from build123d import *

# Parameters (mm, degrees)
SKETCH1_R           = 2.1
BOSS_EXTRUDE1_DEPTH = 50


with BuildPart() as part:
    # Sketch1 → Boss-Extrude1 (new body)
    with BuildSketch(Plane(origin=(0, 0, 0), x_dir=(0, 0, -1), z_dir=(1, 0, 0))):
        with BuildLine():
            Line((-13, 18), (-13, 20))
            Line((-13, 20), (-19, 20))
            ThreePointArc((-19, 20), (-19.707106781, 19.707106781), (-20, 19))
            Line((-20, 19), (-20, 13))
            Line((-20, 13), (-18, 13))
            Line((-18, 13), (-18, 16))
            Line((-18, 16), (-17.060660172, 16))
            Line((-17.060660172, 16), (-14, 12.939339828))
            Line((-14, 12.939339828), (-14, 7.060660172))
            Line((-14, 7.060660172), (-17.060660172, 4))
            Line((-17.060660172, 4), (-18, 4))
            Line((-18, 4), (-18, 7))
            Line((-18, 7), (-20, 7))
            Line((-20, 7), (-20, -7))
            Line((-20, -7), (-18, -7))
            Line((-18, -7), (-18, -4))
            Line((-18, -4), (-17.060660172, -4))
            Line((-17.060660172, -4), (-14, -7.060660172))
            Line((-14, -7.060660172), (-14, -12.939339828))
            Line((-14, -12.939339828), (-17.060660172, -16))
            Line((-17.060660172, -16), (-18, -16))
            Line((-18, -16), (-18, -13))
            Line((-18, -13), (-20, -13))
            Line((-20, -13), (-20, -19))
            ThreePointArc((-20, -19), (-19.707106781, -19.707106781), (-19, -20))
            Line((-19, -20), (-13, -20))
            Line((-13, -20), (-13, -18))
            Line((-13, -18), (-16, -18))
            Line((-16, -18), (-16, -17.060660172))
            Line((-16, -17.060660172), (-12.939339828, -14))
            Line((-12.939339828, -14), (-7.060660172, -14))
            Line((-7.060660172, -14), (-4, -17.060660172))
            Line((-4, -17.060660172), (-4, -18))
            Line((-4, -18), (-7, -18))
            Line((-7, -18), (-7, -20))
            Line((-7, -20), (7, -20))
            Line((7, -20), (7, -18))
            Line((7, -18), (4, -18))
            Line((4, -18), (4, -17.060660172))
            Line((4, -17.060660172), (7.060660172, -14))
            Line((7.060660172, -14), (12.939339828, -14))
            Line((12.939339828, -14), (16, -17.060660172))
            Line((16, -17.060660172), (16, -18))
            Line((16, -18), (13, -18))
            Line((13, -18), (13, -20))
            Line((13, -20), (19, -20))
            ThreePointArc((19, -20), (19.707106781, -19.707106781), (20, -19))
            Line((20, -19), (20, -13))
            Line((20, -13), (18, -13))
            Line((18, -13), (18, -16))
            Line((18, -16), (17.060660172, -16))
            Line((17.060660172, -16), (14, -12.939339828))
            Line((14, -12.939339828), (14, -7.060660172))
            Line((14, -7.060660172), (17.060660172, -4))
            Line((17.060660172, -4), (18, -4))
            Line((18, -4), (18, -7))
            Line((18, -7), (20, -7))
            Line((20, -7), (20, -1))
            ThreePointArc((20, -1), (19.707106781, -0.292893219), (19, 0))
            Line((19, 0), (13, 0))
            Line((13, 0), (13, -2))
            Line((13, -2), (16, -2))
            Line((16, -2), (16, -2.939339828))
            Line((16, -2.939339828), (12.939339828, -6))
            Line((12.939339828, -6), (7.060660172, -6))
            Line((7.060660172, -6), (4, -2.939339828))
            Line((4, -2.939339828), (4, -2))
            Line((4, -2), (7, -2))
            Line((7, -2), (7, 0))
            Line((7, 0), (0.3, 0))
            ThreePointArc((0.3, 0), (0.087867966, 0.087867966), (0, 0.3))
            Line((0, 0.3), (0, 7))
            Line((0, 7), (-2, 7))
            Line((-2, 7), (-2, 4))
            Line((-2, 4), (-2.939339828, 4))
            Line((-2.939339828, 4), (-6, 7.060660172))
            Line((-6, 7.060660172), (-6, 12.939339828))
            Line((-6, 12.939339828), (-2.939339828, 16))
            Line((-2.939339828, 16), (-2, 16))
            Line((-2, 16), (-2, 13))
            Line((-2, 13), (0, 13))
            Line((0, 13), (0, 19))
            ThreePointArc((0, 19), (-0.292893219, 19.707106781), (-1, 20))
            Line((-1, 20), (-7, 20))
            Line((-7, 20), (-7, 18))
            Line((-7, 18), (-4, 18))
            Line((-4, 18), (-4, 17.060660172))
            Line((-4, 17.060660172), (-7.060660172, 14))
            Line((-7.060660172, 14), (-12.939339828, 14))
            Line((-12.939339828, 14), (-16, 17.060660172))
            Line((-16, 17.060660172), (-16, 18))
            Line((-16, 18), (-13, 18))
        make_face()
        with Locations((10, -10)):
            Circle(SKETCH1_R, mode=Mode.SUBTRACT)
        with Locations((-10, 10)):
            Circle(SKETCH1_R, mode=Mode.SUBTRACT)
        Polygon((6, -7.060660172), (-7.060660172, 6), (-12.939339828, 6), (-16.439339828, 2.5), (-18, 2.5), (-18, -2.5), (-16.439339828, -2.5), (-12.5, -6.439339828), (-12.5, -12.5), (-6.439339828, -12.5), (-2.5, -16.439339828), (-2.5, -18), (2.5, -18), (2.5, -16.439339828), (6, -12.939339828), align=None, mode=Mode.SUBTRACT)
    extrude(amount=BOSS_EXTRUDE1_DEPTH)


solid = part.part
The listing builds one solid part. Answer for the finished solid, in the listing's coordinates (mm). A direction names the side the tool comes from. Coordinates: 2 decimals unless noted, no trailing zeros. Order: outer loops, then holes, each group sorted by start corner. A loop starts at its lowest first (then second) coordinate and runs counter-clockwise, first axis right, second up.
Q1. A cutting plane is placed at C-C, the plane z = -10. Write down the section's boundary in (x, y).
Q2. Which of the six approach directions +Z, -Z, +X, -X, +Y, -Y give full straight-line access (tool end or side, diameter ignored) to faces 4 (the face through (25, -4, -20)), 5 (the face through (24.65, 15.51, 14.45)), 6 (the face through (25, -7, -19)), 7 (the face through (25, -7, 19))?
Q3. A cutting plane is placed at B-B, the plane y = -10. Write down the section's boundary in (x, z), and give its area (3 significant figures).
Q4. Given P1, Ø1.8, axis at x = 21.5, z = -10.5, coming from the +Y side; P2, Ø0.6, axis at x = 30, z = 19.5, coming from the +Y side; P3, Ø3.5, axis at x = 18, z = -14.5, coming from the +Y side, each flat-ended and moving along its own axis, determine where each tip first touches the part or whether it passes through.
Q5. For a pull along Y with two mould halves and no side action, classify faces 1 (the face through (25, -1, -7)), 2 (the face through (25, -5, -18)), 3 (the face through (25, -20, 0)) as pulls with the +Y half, pulls with the -Y half, needs draft (parallel to the pull), parting line crosses it, or undercut.
Q6. A cutting plane is placed at D-D, the plane x = 42. State how many separate pieces and enclosed holes the cut face has, and give its area (3 significant figures).
Q7. A cutting plane is placed at A-A, the plane z = 10. Write down the section's boundary in (x, y).
Q8. Consider line 1 (Y direction, x = 26, z = 10); line 2 (Z direction, x = 26.5, y = -9); line 3 (Y direction, x = 19, z = 9.5). Determine where each line is inside the solid, lowest interval first.
Answers follow:
1. outline: (0, -14) - (50, -14) - (50, -12.1) - (0, -12.1) - close; (0, -7.9) - (50, -7.9) - (50, -6) - (0, -6) - close
2. face 4: -Z, +X, -X, +Y, -Y
2. face 5: +X, -X
2. face 6: -Z, +X, -X
2. face 7: +Z, +X, -X
3. outline: (0, -14) - (50, -14) - (50, -12.1) - (0, -12.1) - close; (0, -7.9) - (50, -7.9) - (50, -6) - (0, -6) - close; (0, 12.5) - (50, 12.5) - (50, 14) - (0, 14) - close
3. area: 265 mm2
4. P1: stops at y = -6
4. P2: stops at y = 19.98
4. P3: stops at y = 0
5. face 1: needs draft
5. face 2: undercut
5. face 3: pulls with the -Y half
6. separate pieces: 1
6. enclosed holes: 3
6. area: 423 mm2
7. outline: (0, -14) - (50, -14) - (50, -12.5) - (0, -12.5) - close; (0, 6) - (50, 6) - (50, 7.9) - (0, 7.9) - close; (0, 12.1) - (50, 12.1) - (50, 14) - (0, 14) - close
8. line 1: y = -14 to -12.5, 6 to 7.9, 12.1 to 14
8. line 2: z = -14 to -11.85, -8.15 to -6, 12.5 to 14
8. line 3: y = -14 to -12.5, 6 to 7.96, 12.04 to 14
